Verification items for this drawing (mm, ordinates from the low corner). Give positions to 0.01 mm unless a question says otherwise; leave off trailing zeros. Loops run counter-clockwise (first coordinate to the right, second up) from the corner with the lowest first, then second, coordinate; pieces in that order, holes last. Notation, with made-up numbers: M -23.5,-19.75 L -15.5,-19.75 A22 cw -15.5,-7.75 Z; hole C 67,-26 d4. An arc over 180 degrees is marked long. Write each question's results on one line, items separated by ' | '. Start each with the question number.
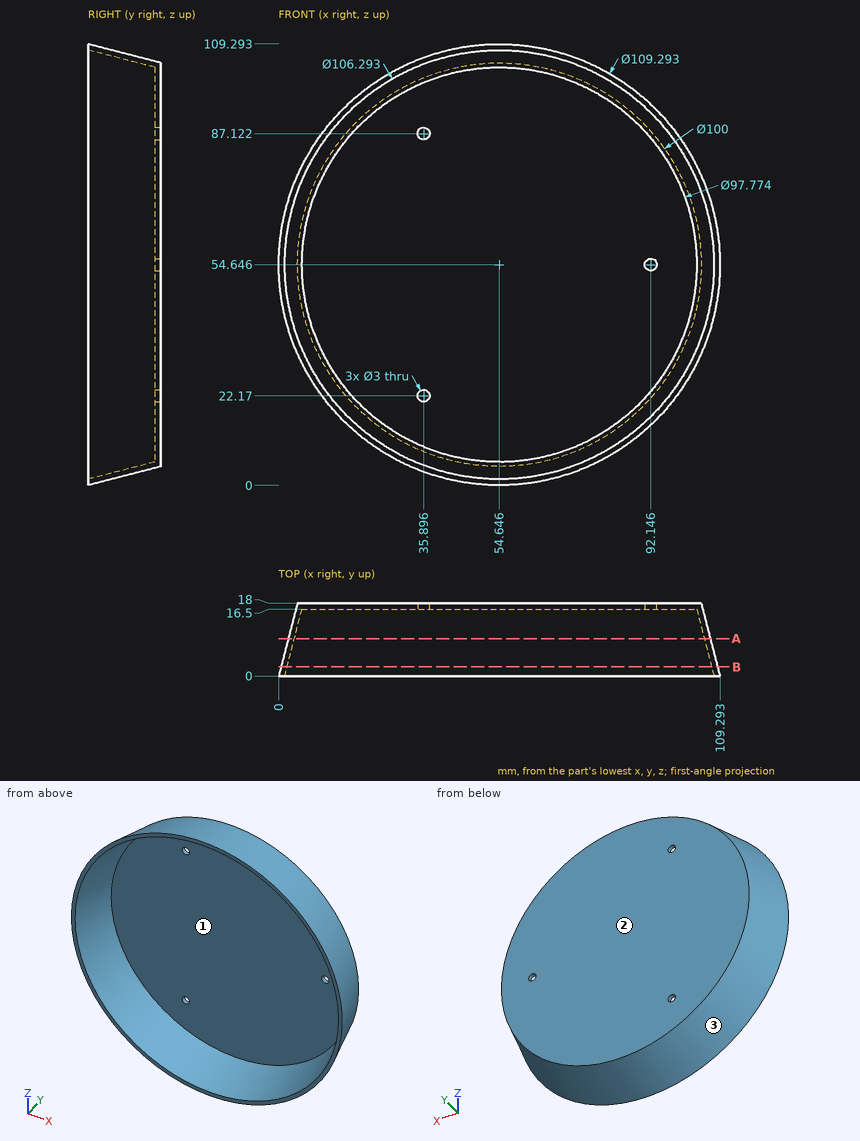
1. Section check B-B, the plane y = 2.25. Record the boundary of the cut face in (x, z) (1 decimal).
2. Thickness scan on probe 1 along Y at (x, z) = (13, 73); probe 2 along Z at (x, y) = (62, 11.5) (1 decimal); probe 3 along Z at (x, y) = (70, 8.75). Record the ranges inside material, lowest first.
3. Section check A-A, the plane y = 9.25. Record the boundary of the cut face in (x, z).
4. Release check for a two-part mould opening along Z. For the marked faces 1, 2 and 3 record: released by +Z, released by -Z, zero draft, split by the parting line, or undercut.
5. Depth check by flat-ended pin: pin 1 Ø3 at (x, y) = (35.5, 14.5) entering from +Z; pin 2 Ø6 at (x, y) = (42, 12.5) entering from -Z; pin 3 Ø1 at (x, z) = (65, 45) entering from -Y; pin 4 Ø2.5 at (x, z) = (35.9, 22.17) entering from +Y. Enter the tip coordinate at first touch or a pass-through.
Filled sheet:
1) outline: C 54.6,54.6 d108.1; hole C 54.6,54.6 d105.1
2) probe 1: 16.5 to 18 | probe 2: 3.5 to 5, 104.3 to 105.8 | probe 3: 4.56 to 6.13, 103.16 to 104.73
3) outline: C 54.65,54.65 d104.52; hole C 54.65,54.65 d101.52
4) face 1: undercut | face 2: zero draft | face 3: split by the parting line
5) pin 1: z = 102.53 | pin 2: z = 3.75 | pin 3: y = 16.5 | pin 4: through
